Verification items for the finished model (mm, model axes). Face numbers are marked on the shaded views. A direction names the side the tool comes from. Round coordinates to 2 decimals unless told otherwise and drop trailing zeros. Order: outer loops, then holes, each group sorted by start corner. A loop starts at its lowest first (then second) coordinate and runs counter-clockwise, first axis right, second up.
```python
from build123d import *

# Parameters (mm, degrees)
BOSS_EXTRUDE1_DEPTH = 50
SKETCH2_R           = 1.25
CUT_EXTRUDE1_DEPTH  = 7
SKETCH3_W           = 8
SKETCH3_H           = 30
SKETCH3_W_2         = 12
SKETCH3_H_2         = 15
CUT_EXTRUDE2_DEPTH  = 2
SKETCH4_R           = 1.5
SKETCH4_W           = 20
SKETCH4_H           = 10
CUT_EXTRUDE3_DEPTH  = 7
FILLET1_R           = 2


with BuildPart() as part:
    # Sketch1 → Boss-Extrude1 (new body)
    with BuildSketch(Plane.XY):
        Polygon((15, 0), (15, -5), (11.45, -5), (11.45, -6), (8.55, -6), (8.55, -5), (5, -5), (5, -2.5), (-15, -2.5), (-15, 0), align=None)
    extrude(amount=BOSS_EXTRUDE1_DEPTH)

    # Sketch2 → Cut-Extrude1 (cut, through all)
    with BuildSketch(Plane(origin=(0, 0, 0), x_dir=(1, 0, 0), z_dir=(0, 1, 0))):
        with Locations((-10.3, -15)):
            Circle(SKETCH2_R)
        with Locations((10.3, -15)):
            Circle(SKETCH2_R)
    extrude(amount=-CUT_EXTRUDE1_DEPTH, mode=Mode.SUBTRACT)

    # Sketch3 → Cut-Extrude2 (cut)
    with BuildSketch(Plane(origin=(0, 0, 0), x_dir=(1, 0, 0), z_dir=(0, 1, 0))):
        with Locations((11, -35)):
            Rectangle(SKETCH3_W, SKETCH3_H)
        with Locations((-9, -30.5)):
            Rectangle(SKETCH3_W_2, SKETCH3_H_2)
    extrude(amount=-CUT_EXTRUDE2_DEPTH, mode=Mode.SUBTRACT)

    # Sketch4 → Cut-Extrude3 (cut, through all)
    with BuildSketch(Plane(origin=(0, -6, 0), x_dir=(-1, 0, 0), z_dir=(0, -1, 0))):
        with Locations((-10, -5)):
            Circle(SKETCH4_R)
        with Locations((5, -5)):
            Rectangle(SKETCH4_W, SKETCH4_H)
    extrude(amount=-CUT_EXTRUDE3_DEPTH, mode=Mode.SUBTRACT)

    # Fillet1
    fillet1_edges = [part.edges().sort_by_distance(p)[0] for p in [
        (5, -2.5, 30),
    ]]
    fillet(fillet1_edges, radius=FILLET1_R)


solid = part.part
```
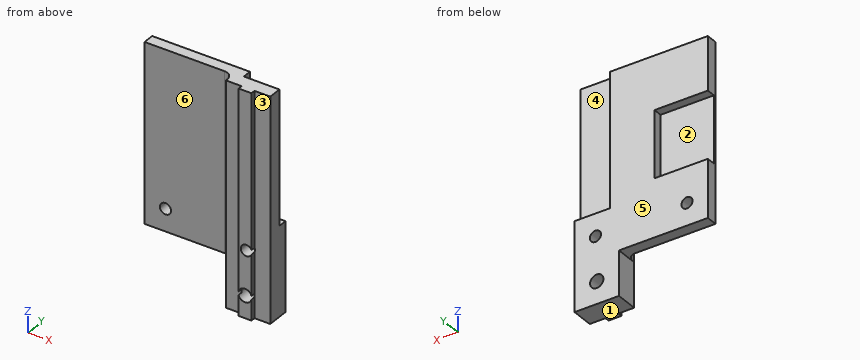
1) Go/stop test with flat-tipped pins: pin 1 Ø1.6 at (x, y) = (-9, -1.5) entering from -Z; pin 2 Ø2 at (x, z) = (-8.5, 22) entering from -Y; pin 3 Ø4 at (x, z) = (6.5, 31.5) entering from -Y. Record where each tip stops, or that it passes through.
2) Tool access check on the marked faces 4, 5 and 6. Record the directions out of +Z, -Z, +X, -X, +Y, -Y that give a thin tool (end or side, any length) a straight path to the whole face; none if there is none.
3) Sectioned sample at B-B on x = -10.3. Record the cut outline in (y, z).
4) Scan lines: probe 1 along X at (y, z) = (-0.55, 15); probe 2 along Y at (x, z) = (1, 37); probe 3 along X at (y, z) = (-1.1, 14.5). Record each from-to range of solid material in increasing order.
5) Sectioned sample at C-C on y = -1.45. Record the cut outline in (x, z), then the cut area to 3 significant figures.
6) Sectioned sample at A-A on z = 15. Record the cut outline in (x, y).
7) Sectioned sample at D-D on z = 32. Record the cut outline in (x, y), then the cut area to 3 significant figures.
8) Draft check along Z on the marked faces 1, 2 and 3. Enter one of: released by +Z, released by -Z, zero draft, split by the parting line, or undercut.
Returned:
1. pin 1: stops at z = 10
1. pin 2: stops at y = -2.5
1. pin 3: stops at y = -5
2. face 4: +Z, +X, +Y
2. face 5: +Z, -Z, +X, -X, +Y
2. face 6: +Z, -Z, -X, -Y
3. outline: (-2.5, 10) - (0, 10) - (0, 13.75) - (-2.5, 13.75) - close; (-2.5, 16.25) - (0, 16.25) - (0, 23) - (-2, 23) - (-2, 38) - (0, 38) - (0, 50) - (-2.5, 50) - close
4. probe 1: x = -15 to -11.55, -9.05 to 9.05, 11.55 to 15
4. probe 2: y = -2.5 to 0
4. probe 3: x = -15 to -11.45, -9.15 to 9.15, 11.45 to 15
5. outline: (-15, 10) - (5, 10) - (5, 0) - (15, 0) - (15, 20) - (7, 20) - (7, 50) - (-15, 50) - (-15, 38) - (-3, 38) - (-3, 23) - (-15, 23) - close; hole circle Ø2.5 at (-10.3, 15); hole circle Ø3 at (10, 5); hole circle Ø2.5 at (10.3, 15)
5. area: 863 mm2
6. outline: (-15, -2.5) - (-11.55, -2.5) - (-11.55, 0) - (-15, 0) - close; (-9.05, -2.5) - (3, -2.5) arc R2 cw to (5, -4.5) - (5, -5) - (8.55, -5) - (8.55, -6) - (9.05, -6) - (9.05, 0) - (-9.05, 0) - close; (11.55, -5) - (15, -5) - (15, 0) - (11.55, 0) - close
7. outline: (-15, -2.5) - (3, -2.5) arc R2 cw to (5, -4.5) - (5, -5) - (8.55, -5) - (8.55, -6) - (11.45, -6) - (11.45, -5) - (15, -5) - (15, -2) - (7, -2) - (7, 0) - (-3, 0) - (-3, -2) - (-15, -2) - close
7. area: 63.8 mm2
8. face 1: released by -Z
8. face 2: undercut
8. face 3: zero draft
